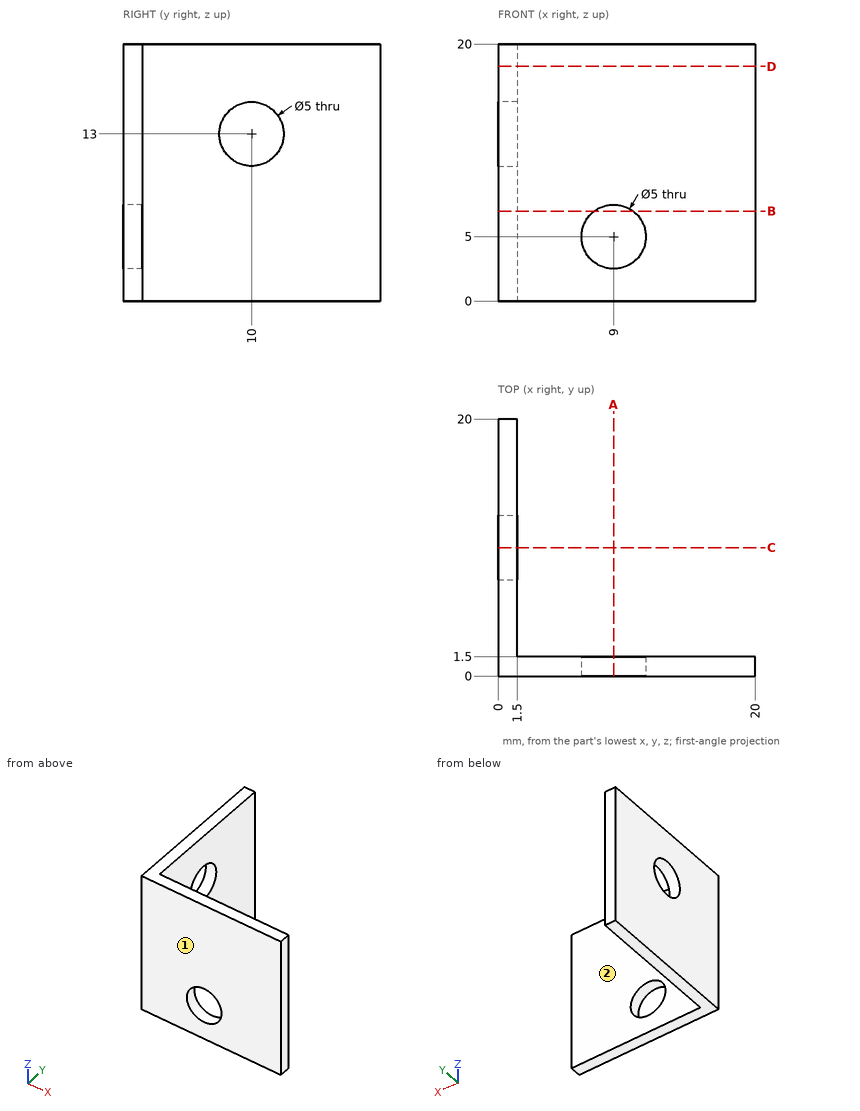
For this review, use the dimensioned drawing (mm, ordinates from the lowest corner) and the shaded views. A direction names the side the tool comes from. Round coordinates to 2 decimals unless told otherwise and drop trailing zeros. Loops run counter-clockwise (first coordinate to the right, second up) from the corner with the lowest first, then second, coordinate; pieces in that order, holes last. Notation, with made-up numbers: M 75,-23 L 102,-23 A13 ccw 102,2 Z; hole C 65.5,54.5 d10. An arc over 180 degrees is marked long. Answer as CSV lines item,"result".
1. We need section C-C (y = 10). Give the boundary of the cut face in (x, z), plus the area to 3 significant figures.
Outcome:
outline,"M 0,0 L 1.5,0 L 1.5,10.5 L 0,10.5 Z; M 0,15.5 L 1.5,15.5 L 1.5,20 L 0,20 Z"
area,"22.5 mm2"
2. We need section A-A (x = 9). Give the boundary of the cut face in (y, z).
Outcome:
outline,"M 0,0 L 1.5,0 L 1.5,2.5 L 0,2.5 Z; M 0,7.5 L 1.5,7.5 L 1.5,20 L 0,20 Z"
3. To check wall thickness, follow L1, parallel to Y at x = 1, z = 13; L2, parallel to X at y = 7, z = 15.25. State the ranges of each line that lie inside material, in increasing order. Write a range as [from, to].
Outcome:
L1,"y = [0, 7.5], [12.5, 20]"
L2,"x = [0, 1.5]"
4. We need section B-B (z = 7). Give the boundary of the cut face in (x, y), plus the area to 4 significant figures.
Outcome:
outline,"M 0,0 L 7.5,0 L 7.5,1.5 L 1.5,1.5 L 1.5,20 L 0,20 Z; M 10.5,0 L 20,0 L 20,1.5 L 10.5,1.5 Z"
area,"53.25 mm2"
5. Insertion check: pin 1 Ø5.5 at (x, z) = (8.5, 12.5) entering from +Y; pin 2 Ø6.5 at (y, z) = (10, 13) entering from +X. Each pin has a flat end and moves straight along its axis. Give the tip position at first contact, or say it passes through.
Outcome:
pin 1,"stops at y = 1.5"
pin 2,"stops at x = 1.5"
6. We need section D-D (z = 18.25). Give the boundary of the cut face in (x, y).
Outcome:
outline,"M 0,0 L 20,0 L 20,1.5 L 1.5,1.5 L 1.5,20 L 0,20 Z"
7. For the marked faces 1 and 2, list the 3-axis set-ups (+Z, -Z, +X, -X, +Y, -Y) from which the entire face can be reached by the end or side of a thin tool; tool diameter is ignored.
Outcome:
face 1,"+Z, -Z, +X, -X, -Y"
face 2,"+Z, -Z, +X, +Y"
